Autodesk Inventor part; units mm, degrees
ref_plane "YZ Plane" through (0, 0, 0) normal (1, 0, 0) x (0, 1, 0)
ref_plane "XZ Plane" through (0, 0, 0) normal (0, 1, 0) x (-1, 0, 0)
ref_plane "XY Plane" through (0, 0, 0) normal (0, 0, 1) x (1, 0, 0)
sketch "Sketch1" plane through (0, 0, 0) normal (0, 0, 1) x (1, 0, 0)
  line L0 (333.7348, 101.6) -> (333.7348, 584.2)
  line L1 (92.4348, 101.6) -> (92.4348, 368.3)
  line L2 (92.4348, 368.3) -> (301.9848, 368.3)
  line L3 (301.9848, 368.3) -> (301.9848, 101.6)
  line L4 (301.9848, 101.6) -> (333.7348, 101.6)
  line L5 (92.4348, 101.6) -> (60.6848, 101.6)
  line L6 (60.6848, 101.6) -> (60.6848, 584.2)
  line L7 (60.6848, 584.2) -> (333.7348, 584.2)
  point P0 (0, 0)
  point P1 (197.2098, 254)
  point P2 (197.2098, 391.541)
  point P3 (78.0958, 322.7705)
  point P4 (78.0958, 185.2295)
  point P5 (197.2098, 116.459)
  point P6 (316.3238, 185.2295)
  point P7 (316.3238, 322.7705)
  point P8 (187.6848, 546.1)
  point P9 (311.5098, 254)
  point P10 (311.5098, 558.8)
  point P11 (311.5098, 431.8)
  point P12 (82.9098, 558.8)
  point P13 (82.9098, 431.8)
  point P14 (82.9098, 254)
  point P15 (235.3098, 431.8)
  point P16 (159.1098, 431.8)
  dimension "d1" = 482.6
  dimension "d4" = 137.541
  dimension "d7" = 360
  dimension "d9" = 31.75
  dimension "d21" = 31.75
  dimension "d23" = 114.3
  dimension "d24" = 38.1
  dimension "d33" = 273.05
  dimension "d34" = 146.05
  dimension "d35" = 25.4
  dimension "d36" = 25.4
  dimension "d39" = 177.8
  dimension "d40" = 177.8
  dimension "d48" = 22.225
  dimension "d49" = 22.225
  dimension "d51" = 76.2
  dimension "d52" = 76.2
  dimension "d53" = 76.2
  dimension "d54" = 209.55
  dimension "d55" = 266.7
  dimension "d56" = 104.775
  dimension "d57" = 152.4
  dimension "d58" = 152.4
extrude "Extrusion1" add sketch "Sketch1" against normal blind 3.175
hole "Hole1" at (197.2098, 254, 0) at (197.2098, 391.541, 0) at (78.0958, 322.7705, 0) at (78.0958, 185.2295, 0) at (197.2098, 116.459, 0) at (316.3238, 185.2295, 0) at (316.3238, 322.7705, 0) direction (0, 0, -1) diameter 6.35 depth 25.4 tip angle 118
hole "Hole2" at (187.6848, 546.1, 0) direction (0, 0, -1) diameter 12.7 depth 25.4 tip angle 118
hole "Hole3" at (311.5098, 254, 0) at (311.5098, 558.8, 0) at (311.5098, 431.8, 0) at (82.9098, 558.8, 0) at (82.9098, 431.8, 0) at (82.9098, 254, 0) at (159.1098, 431.8, 0) at (235.3098, 431.8, 0) direction (0, 0, -1) diameter 6.35 depth 25.4 tip angle 118
properties part number "bottom plate"
Read the model definition and answer for the solid it produces. Units are mm, in the model's axes. Round coordinates to 2 decimals unless told otherwise and drop trailing zeros. Order: outer loops, then holes, each group sorted by start corner. A loop starts at its lowest first (then second) coordinate and runs counter-clockwise, first axis right, second up.
1) The part is cut by section C-C on y = 546.1. Write down the section's boundary in (x, z) (3 decimals).
2) The part is cut by section A-A on y = 230. Write down the section's boundary in (x, z) (3 decimals), plus the area to 3 significant figures.
3) The part is cut by section B-B on z = -0.85. Give the number of separate pieces and of enclosed holes in the cut face, plus the area to 3 significant figures.
4) Flat-ended cylindrical pins translate along their axes: pin 1 (8 mm diameter, centred on x = 296, y = 309, fed in from -Z); pin 2 (1.6 mm diameter, centred on x = 175, z = -2.5, fed in from -Y). Find the tip coordinate at first contact, or state that the pin passes through.
5) Straight lines are drawn through the part: L1, parallel to X at y = 254, z = -1.1; L2, parallel to X at y = 431.5, z = -0.45; L3, parallel to X at y = 342, z = -1.2. For each, find the intervals that lie inside material, in ascending order.
6) The mould has two halves that part along X. Classify faces 1 (the face through (185.777, 540.043, -1.61)), 2 (the face through (195, 454, -3.175)): released by +X, released by -X, zero draft, split by the parting line, or undercut.
7) The part is cut by section D-D on x = 277. Write down the section's boundary in (y, z) (3 decimals), plus the area to 3 significant figures.
Resolved:
1. outline: (60.685, -3.175) - (181.335, -3.175) - (181.335, 0) - (60.685, 0) - close; (194.035, -3.175) - (333.735, -3.175) - (333.735, 0) - (194.035, 0) - close
2. outline: (60.685, -3.175) - (92.435, -3.175) - (92.435, 0) - (60.685, 0) - close; (301.985, -3.175) - (333.735, -3.175) - (333.735, 0) - (301.985, 0) - close
2. area: 202 mm2
3. separate pieces: 1
3. enclosed holes: 14
3. area: 75,300 mm2
4. pin 1: passes through
4. pin 2: stops at y = 368.3
5. L1: x = 60.68 to 79.73, 86.08 to 92.43, 301.98 to 308.33, 314.68 to 333.73
5. L2: x = 60.68 to 79.75, 86.07 to 155.95, 162.27 to 232.15, 238.47 to 308.35, 314.67 to 333.73
5. L3: x = 60.68 to 92.43, 301.98 to 333.73
6. face 1: undercut
6. face 2: zero draft
7. outline: (368.3, -3.175) - (584.2, -3.175) - (584.2, 0) - (368.3, 0) - close
7. area: 685 mm2
